from build123d import *

# Parameters (mm, degrees)
F1_DEPTH = 12.7
F2_D     = 10.0838
F3_W     = 38.1
F3_H     = 12.7
F4_DEPTH = 12.7


with BuildPart() as f1:
    # F0 (on Front) → F1 (new body)
    with BuildSketch(Plane.XZ):
        Polygon((0, 288.925), (0, 0), (336.55, 0), (336.55, 187.325), (234.95, 288.925), align=None)
    extrude(amount=F1_DEPTH)

    # F2 (through all)
    with Locations(Plane(origin=(0, 0, 0), x_dir=(1, 0, 0), z_dir=(0, 1, 0))):
        with Locations((311.15, -28.575), (168.275, -28.575), (25.4, -28.575), (25.4, -260.35), (209.55, -260.35), (117.475, -260.35)):
            Hole(F2_D / 2)

    # F3 (on face) → F4 (join)
    with BuildSketch(Plane.XZ.offset(12.7)):
        with Locations((58.7375, 295.275)):
            Rectangle(F3_W, F3_H)
        with Locations((176.2125, 295.275)):
            Rectangle(F3_W, F3_H)
        with Locations((84.1375, -6.35)):
            Rectangle(F3_W, F3_H)
        with Locations((252.4125, -6.35)):
            Rectangle(F3_W, F3_H)
    extrude(amount=-F4_DEPTH)


solid = f1.part
Design review of the part built by this model. Coordinates are the model's own, in mm. A direction names the side the tool comes from. Coordinates: 2 decimals unless noted, no trailing zeros. Order: outer loops, then holes, each group sorted by start corner. A loop starts at its lowest first (then second) coordinate and runs counter-clockwise, first axis right, second up. Notation, with made-up numbers: M 48,-16 L 87,-16 A33 cw 87,23 Z; hole C -0.75,14 d6. An arc over 180 degrees is marked long. Use a Markdown table: item, result.
(1) For faces 5 (the flat face through (39.688, -6, 295)), 6 (the flat face through (304, -6, 0)), 7 (the flat face through (167, -6, 0)), 8 (the flat face through (195.263, -6, 295)), 9 (the flat face through (118, -6, 288.925)), list the 3-axis set-ups (+Z, -Z, +X, -X, +Y, -Y) from which the entire face can be reached by the end or side of a thin tool; tool diameter is ignored.
Worked answers:
| item | result |
|---|---|
| face 5 | +Z, -X, +Y, -Y |
| face 6 | -Z, +X, +Y, -Y |
| face 7 | -Z, +Y, -Y |
| face 8 | +Z, +X, +Y, -Y |
| face 9 | +Z, +Y, -Y |
(2) Add section D-D (y = -8). Count the separate pieces of the cut face and the enclosed holes in it, then the cut area to 3 significant figures.
Worked answers:
| item | result |
|---|---|
| separate pieces | 1 |
| enclosed holes | 6 |
| area | 93,500 mm2 |
(3) Draft analysis for pull direction Z (two halves, no side actions). For faces 1 (the flat face through (84, -6, -12.7)), 2 (the cylindrical face through (173.31, -6.44, 28.35)), 3 (the flat face through (215, -6, 288.925)), 4 (the cylindrical face through (22.69, -6.439, 24.324)), state which applies: released by +Z, released by -Z, zero draft, split by the parting line, or undercut.
Worked answers:
| item | result |
|---|---|
| face 1 | released by -Z |
| face 2 | undercut |
| face 3 | released by +Z |
| face 4 | undercut |
(4) Add section B-B (z = 260.35). Give the boundary of the cut face in (x, y) (3 decimals).
Worked answers:
| item | result |
|---|---|
| outline | M 0,-12.7 L 20.358,-12.7 L 20.358,0 L 0,0 Z; M 30.442,-12.7 L 112.433,-12.7 L 112.433,0 L 30.442,0 Z; M 122.517,-12.7 L 204.508,-12.7 L 204.508,0 L 122.517,0 Z; M 214.592,-12.7 L 263.525,-12.7 L 263.525,0 L 214.592,0 Z |
(5) Add section A-A (x = 209.55). Give the boundary of the cut face in (y, z) (3 decimals), then the cut area to 3 significant figures.
Worked answers:
| item | result |
|---|---|
| outline | M -12.7,0 L 0,0 L 0,255.308 L -12.7,255.308 Z; M -12.7,265.392 L 0,265.392 L 0,288.925 L -12.7,288.925 Z |
| area | 3,540 mm2 |
(6) Wall thickness on probe 1 along Z at (x, y) = (25.4, -4) (3 decimals); probe 2 along X at (y, z) = (-5, 27); probe 3 along X at (y, z) = (-6.5, 260.35) (3 decimals): over which ranges is each line inside the solid? List them lowest first.
Worked answers:
| item | result |
|---|---|
| probe 1 | z = 0 to 23.533, 33.617 to 255.308, 265.392 to 288.925 |
| probe 2 | x = 0 to 20.61, 30.19 to 163.49, 173.06 to 306.36, 315.94 to 336.55 |
| probe 3 | x = 0 to 20.358, 30.442 to 112.433, 122.517 to 204.508, 214.592 to 263.525 |
(7) Add section C-C (x = 25.4). Give the boundary of the cut face in (y, z) (3 decimals), then the cut area to 3 significant figures.
Worked answers:
| item | result |
|---|---|
| outline | M -12.7,0 L 0,0 L 0,23.533 L -12.7,23.533 Z; M -12.7,33.617 L 0,33.617 L 0,255.308 L -12.7,255.308 Z; M -12.7,265.392 L 0,265.392 L 0,288.925 L -12.7,288.925 Z |
| area | 3,410 mm2 |
(8) For P1, Ø6.5, axis at x = 24, y = -3.5, coming from the +Z side (3 decimals); P2, Ø6.5, axis at x = 155, y = -5, coming from the -Z side; P3, Ø4, axis at y = -6, z = -5.5, coming from the +X side, all flat-tipped, find the tip position at first contact; note any pin that passes through.
Worked answers:
| item | result |
|---|---|
| P1 | stops at z = 288.925 |
| P2 | stops at z = 0 |
| P3 | stops at x = 271.46 |
